The listing builds one solid part. Answer for the finished solid, in the listing's coordinates (mm). A direction names the side the tool comes from. Coordinates: 2 decimals unless noted, no trailing zeros. Order: outer loops, then holes, each group sorted by start corner. A loop starts at its lowest first (then second) coordinate and runs counter-clockwise, first axis right, second up. Notation, with made-up numbers: (-27, -11) -> (-5, -11) arc R16 cw to (-5, 8) -> close; hole circle Ø11 at (-31, -6). An arc over 180 degrees is marked (long way). Write each question's results on one line, items separated by ' | '. Start each with the question number.
(1) Determine the mould class of faces 4 (the face through (0, 1, -36)), 5 (the face through (-1, 3, -1)), 6 (the face through (1, 1, -40)), 7 (the face through (50, 1, 40)) for opening direction Z: +Z half, -Z half, draft (parallel to the pull), parting line (faces both ways), or undercut.
(2) Straight lines are drawn through the part: L1, parallel to X at y = 2.3, z = -33; L2, parallel to Z at x = -69.5, y = 1.7; L3, parallel to X at y = 1.6, z = 33. For each, find the intervals that lie inside material, in ascending order.
(3) The part is cut by section B-B, the plane x = -69.5. Give the vertices of the cut face in (y, z).
(4) A tool of negligible diameter and unlimited length cuts with its end or side. For faces 1 (the face through (46, 1, 17)), 2 (the face through (-72.5, 1, -1)), 3 (the face through (28, 1, 20)), from which of +Z, -Z, +X, -X, +Y, -Y can it reach the whole face along a straight path? Write none if from no direction.
(5) The part is cut by section C-C, the plane z = 15. Give the vertices of the cut face in (x, y), then the cut area to 3 significant figures.
(6) Given pin 1 (1 mm diameter, centred on x = 26.5, y = 2, fed in from +Z), flat-ended and moving along its own axis, determine where the tip first touches the part or whether it passes through.
(7) The part is cut by section A-A, the plane z = -33. Give the vertices of the cut face in (x, y).
(8) The part is cut by section D-D, the plane z = 33. Give the vertices of the cut face in (x, y), then the cut area to 3 significant figures.
```python
from build123d import *

# Parameters (mm, degrees)
SKETCH1_R           = 1.5
SKETCH1_W           = 3
SKETCH1_H           = 7
SKETCH1_W_2         = 4
SKETCH1_H_2         = 3
BOSS_EXTRUDE1_DEPTH = 3


with BuildPart() as part:
    # Sketch1 → Boss-Extrude1 (new body)
    with BuildSketch(Plane(origin=(0, 0, 0), x_dir=(1, 0, 0), z_dir=(0, 1, 0))):
        Polygon((-72.5, -40), (-28, -40), (-28, 0), (28, 0), (28, -40), (72.5, -40), (72.5, 40), (-72.5, 40), align=None)
        with Locations(Location((-69.5, 33, 0), (0, 0, 270))):
            Circle(SKETCH1_R, mode=Mode.SUBTRACT)
        with Locations(Location((-43.5, 33, 0), (0, 0, 270))):
            Circle(SKETCH1_R, mode=Mode.SUBTRACT)
        with Locations(Location((-43.5, -33, 0), (0, 0, 270))):
            Circle(SKETCH1_R, mode=Mode.SUBTRACT)
        with Locations(Location((-69.5, -33, 0), (0, 0, 270))):
            Circle(SKETCH1_R, mode=Mode.SUBTRACT)
        with Locations((46, 5.5)):
            Rectangle(SKETCH1_W, SKETCH1_H, mode=Mode.SUBTRACT)
        with Locations((46, 18.5)):
            Rectangle(SKETCH1_W, SKETCH1_H, mode=Mode.SUBTRACT)
        with Locations((46, -7.5)):
            Rectangle(SKETCH1_W, SKETCH1_H, mode=Mode.SUBTRACT)
        with Locations((46, -20.5)):
            Rectangle(SKETCH1_W, SKETCH1_H, mode=Mode.SUBTRACT)
        with Locations((46, -33.5)):
            Rectangle(SKETCH1_W, SKETCH1_H, mode=Mode.SUBTRACT)
        with Locations((0, 37.5)):
            Rectangle(SKETCH1_W_2, SKETCH1_H_2, mode=Mode.SUBTRACT)
        with Locations((8, 37.5)):
            Rectangle(SKETCH1_W_2, SKETCH1_H_2, mode=Mode.SUBTRACT)
        with Locations((16, 37.5)):
            Rectangle(SKETCH1_W_2, SKETCH1_H_2, mode=Mode.SUBTRACT)
    extrude(amount=BOSS_EXTRUDE1_DEPTH)


solid = part.part
```
Established:
1) face 4: undercut | face 5: draft | face 6: -Z half | face 7: +Z half
2) L1: x = -72.5 to -71, -68 to -45, -42 to 72.5 | L2: z = -40 to -34.5, -31.5 to 31.5, 34.5 to 40 | L3: x = -72.5 to -71, -68 to -45, -42 to -28, 28 to 44.5, 47.5 to 72.5
3) outline: (0, -40) -> (3, -40) -> (3, -34.5) -> (0, -34.5) -> close; (0, -31.5) -> (3, -31.5) -> (3, 31.5) -> (0, 31.5) -> close; (0, 34.5) -> (3, 34.5) -> (3, 40) -> (0, 40) -> close
4) face 1: +Y, -Y | face 2: +Z, -Z, -X, +Y, -Y | face 3: +Z, +Y, -Y
5) outline: (-72.5, 0) -> (-28, 0) -> (-28, 3) -> (-72.5, 3) -> close; (28, 0) -> (72.5, 0) -> (72.5, 3) -> (28, 3) -> close | area: 267 mm^2
6) pin 1: stops at z = 0
7) outline: (-72.5, 0) -> (-71, 0) -> (-71, 3) -> (-72.5, 3) -> close; (-68, 0) -> (-45, 0) -> (-45, 3) -> (-68, 3) -> close; (-42, 0) -> (72.5, 0) -> (72.5, 3) -> (-42, 3) -> close
8) outline: (-72.5, 0) -> (-71, 0) -> (-71, 3) -> (-72.5, 3) -> close; (-68, 0) -> (-45, 0) -> (-45, 3) -> (-68, 3) -> close; (-42, 0) -> (-28, 0) -> (-28, 3) -> (-42, 3) -> close; (28, 0) -> (44.5, 0) -> (44.5, 3) -> (28, 3) -> close; (47.5, 0) -> (72.5, 0) -> (72.5, 3) -> (47.5, 3) -> close | area: 240 mm^2
